The model under review builds one solid part; all positions refer to its coordinate system, in mm. A direction names the side the tool comes from. Coordinates: 2 decimals unless noted, no trailing zeros. Order: outer loops, then holes, each group sorted by start corner. A loop starts at its lowest first (then second) coordinate and runs counter-clockwise, first axis right, second up.
Autodesk Inventor part; units mm, degrees
ref_plane "Work Plane1" through (0, 0, 0) normal (1, 0, 0) x (0, 1, 0)
ref_plane "XZ Plane" through (0, 0, 0) normal (0, 1, 0) x (-1, 0, 0)
ref_plane "XY Plane" through (0, 0, 0) normal (0, 0, 1) x (1, 0, 0)
sketch "Sketch1" plane through (0, 0, 0) normal (0, 0, 1) x (1, 0, 0)
  circle A0 centre (0, 0) radius 3.45
  circle A1 centre (0, 0) radius 2.05
  line L0 (-2.59, 0) -> (2.59, 0) construction
  line L1 (0, -2.59) -> (0, 2.59) construction
  dimension "d0" = 6.9
  dimension "d1" = 4.1
extrude "Выдавливание1" add sketch "Sketch1" along normal blind 1
sketch "Sketch2" plane through (0, 0, 0) normal (0, 1, 0) x (-1, 0, 0)
  line L0 (-2.05, 1) -> (2.05, 1) construction
  line L1 (2.05, 0) -> (-2.05, 0) construction
  line L2 (-0.432, 1) -> (-0.068, 0)
  line L3 (0.068, 1) -> (0.432, 0)
  line L4 (0, 0.5) -> (-0.182, 1) construction
  line L5 (0, 0) -> (0, 1) construction
  line L6 (-0.432, 1) -> (0.068, 1)
  line L7 (-0.068, 0) -> (0.432, 0)
  dimension "d4" = 70
  dimension "d13" = 0.5
extrude "Выдавливание2" cut sketch "Sketch2" along normal through all
ref_plane "Work Plane1" through (0, 0, 0) normal (1, 0, 0) x (0, 1, 0)
equation "\"d0\" = d + 2 * b"
equation "\"d1\" = d"
equation "\"d2\" = s_"
equation "\"d4\" = Angle"
equation "\"d13\" = 0.5 * s_"
equation "\"d7\" = s_"
equation "\"ND\" = 4"
equation "\"d\" = 4.1"
equation "\"b\" = 1.4"
equation "\"s_\" = 1"
equation "\"D_\" = 6.9"
equation "\"Angle\" = 70deg"
properties part number "Шайба У 4Л ГОСТ 6402-78" material "Сталь, мягкая"
(1) Wall thickness on probe 1 along X at (y, z) = (0, 0.4); probe 2 along X at (y, z) = (3, 0.15); probe 3 along Y at (x, z) = (0, 0.5): over which ranges is each line inside the solid? List them lowest first.
A:
probe 1: x = -3.45 to -2.05, 2.05 to 3.45
probe 2: x = -1.7 to -0.38, 0.12 to 1.7
probe 3: y = -3.45 to -2.05
(2) We need section A-A, the plane y = 0.5. Write out the cut boundary in (x, z).
A:
outline: (-3.41, 0) - (-1.99, 0) - (-1.99, 1) - (-3.41, 1) - close; (1.99, 0) - (3.41, 0) - (3.41, 1) - (1.99, 1) - close
(3) We need section D-D, the plane x = -2.5. Write out the cut boundary in (y, z), and give its area (4 significant figures).
A:
outline: (-2.38, 0) - (2.38, 0) - (2.38, 1) - (-2.38, 1) - close
area: 4.755 mm2
(4) We need section B-B, the plane x = -1.5. Write out the cut boundary in (y, z).
A:
outline: (-3.11, 0) - (-1.4, 0) - (-1.4, 1) - (-3.11, 1) - close; (1.4, 0) - (3.11, 0) - (3.11, 1) - (1.4, 1) - close
(5) Machinability: for faces 1 (the face through (0.253, 2.717, 0.507)), 2 (the face through (0, -2.3, 0)), which of the approach directions +Z, -Z, +X, -X, +Y, -Y give a long, thin tool a straight path to every point of the face, cutting with its end or side? Answer none if there is none.
A:
face 1: +Z, +Y
face 2: -Z, +X, -X, +Y, -Y
(6) Draft analysis for pull direction X (two halves, no side actions). For faces 3 (the face through (-0.247, 2.717, 0.507)), 4 (the face through (0, -2.3, 1)), state which applies: released by +X, released by -X, zero draft, split by the parting line, or undercut.
A:
face 3: undercut
face 4: zero draft
(7) We need section C-C, the plane z = 0.2. Write out the cut boundary in (x, y).
A:
outline: (-0.36, 2.02) - (-0.36, 3.43) arc R3.45 ccw (long way) to (0.14, 3.45) - (0.14, 2.05) arc R2.05 cw (long way) to start
